Geometry check sheet. Reference: drawing and pictorial views, mm from the part's lowest x, y, z. A direction names the side the tool comes from. Round coordinates to 2 decimals unless told otherwise and drop trailing zeros. Order: outer loops, then holes, each group sorted by start corner. A loop starts at its lowest first (then second) coordinate and runs counter-clockwise, first axis right, second up.
(1) Sectioned sample at D-D (y = 23). Record the boundary of the cut face in (x, z) (1 decimal).
(2) Go/stop test with flat-tipped pins: pin 1 (3 mm diameter, centred on y = 28, z = 73, fed in from -X); pin 2 (6 mm diameter, centred on x = 32.5, y = 11, fed in from -Z); pin 3 (4 mm diameter, centred on x = 43, y = 6.5, fed in from -Z). Record where each tip stops, or that it passes through.
(3) Material ranges on line 1 along Y through (x, z) = (35, 19.5) (1 decimal); line 2 along Z through (x, y) = (36.5, 27) (1 decimal); line 3 along X through (y, z) = (24, 77.5) (1 decimal), recorded low to high.
(4) Set-up check for the marked faces 1, 2 and 3: record each of +Z, -Z, +X, -X, +Y, -Y from which the full face is reachable in a straight line by a thin tool's end or side.
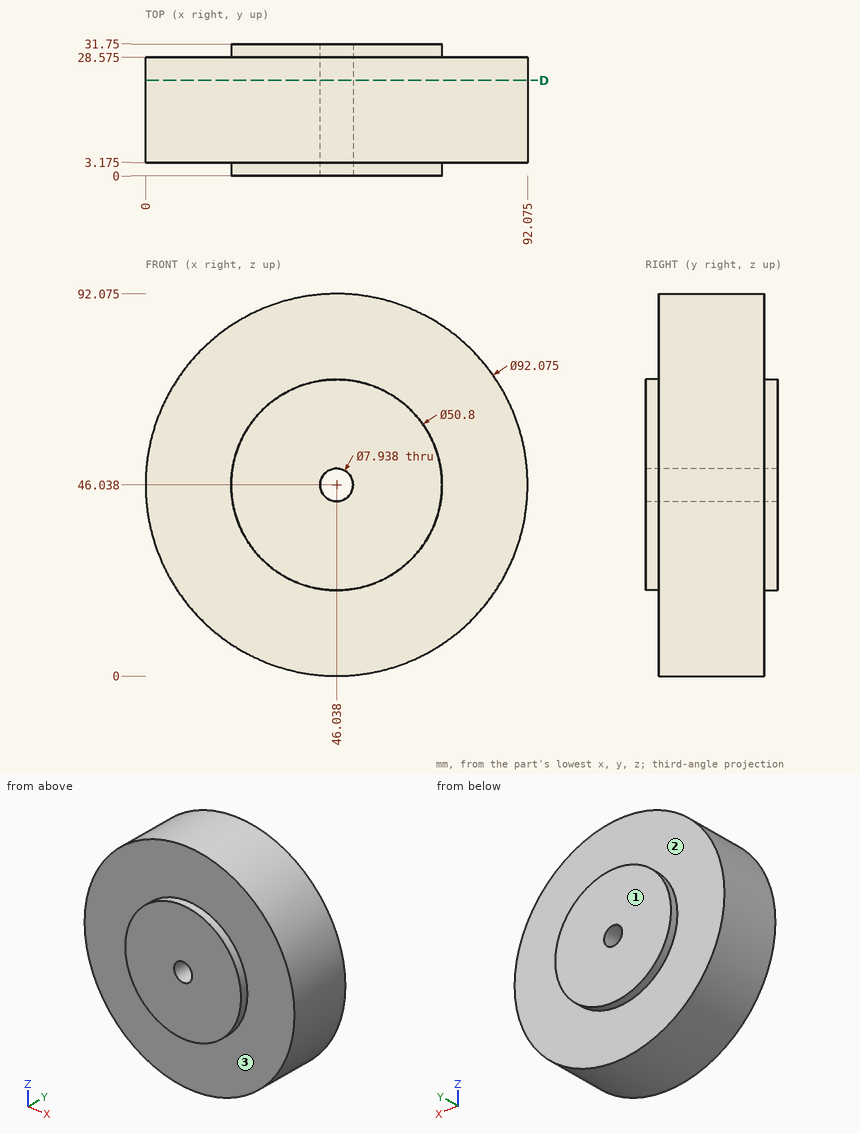
Answer below:
1. outline: circle Ø92.1 at (46, 46); hole circle Ø7.9 at (46, 46)
2. pin 1: stops at x = 7.68
2. pin 2: stops at z = 1.22
2. pin 3: stops at z = 0.01
3. line 1: y = 3.2 to 28.6
3. line 2: z = 1 to 91.1
3. line 3: x = 12.4 to 79.6
4. face 1: +Z, -Z, +X, -X, +Y
4. face 2: +Y
4. face 3: -Y
